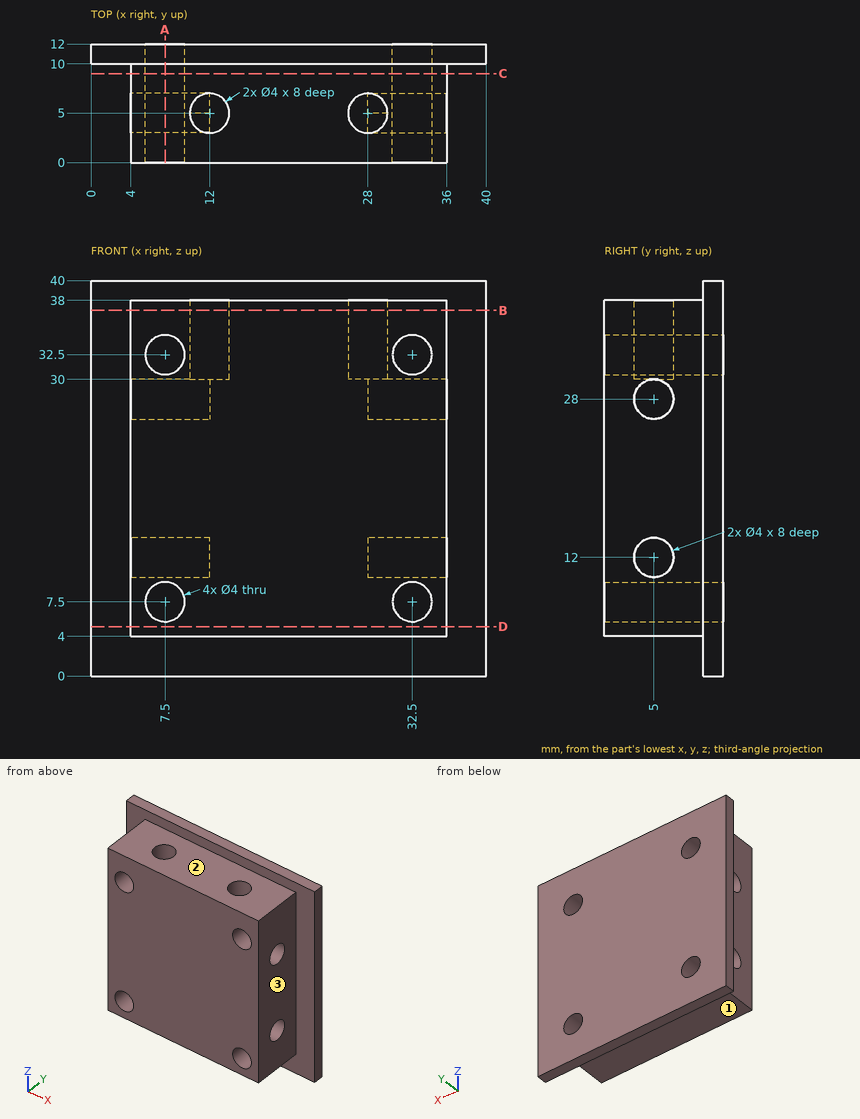
Design review of the part shown in the three views and the two pictorial views. Dimensions are in mm from the part's minimum x, y and z. A direction names the side the tool comes from. Round coordinates to 2 decimals unless told otherwise and drop trailing zeros. Loops run counter-clockwise (first coordinate to the right, second up) from the corner with the lowest first, then second, coordinate; pieces in that order, holes last.
Q1. Insertion check: pin 1 Ø3 at (y, z) = (3.5, 29) entering from +X; pin 2 Ø6 at (x, y) = (23.5, 6) entering from -Z; pin 3 Ø3 at (x, y) = (22, 7) entering from +Z. Each pin has a flat end and moves straight along its axis. Give the tip position at first contact, or say it passes through.
Result sheet:
pin 1: stops at x = 36
pin 2: stops at z = 4
pin 3: stops at z = 38
Q2. Add section C-C on y = 9. Write out the cut boundary in (x, z), plus the area to 3 significant figures.
Result sheet:
outline: (4, 4) - (36, 4) - (36, 38) - (4, 38) - close; hole circle Ø4 at (7.5, 7.5); hole circle Ø4 at (7.5, 32.5); hole circle Ø4 at (32.5, 7.5); hole circle Ø4 at (32.5, 32.5)
area: 1,040 mm2
Q3. Add section B-B on z = 37. Write out the cut boundary in (x, y).
Result sheet:
outline: (0, 10) - (4, 10) - (4, 0) - (36, 0) - (36, 10) - (40, 10) - (40, 12) - (0, 12) - close; hole circle Ø4 at (12, 5); hole circle Ø4 at (28, 5)
Q4. Add section D-D on z = 5. Write out the cut boundary in (x, y), plus the area to 3 significant figures.
Result sheet:
outline: (0, 10) - (4, 10) - (4, 0) - (36, 0) - (36, 10) - (40, 10) - (40, 12) - (0, 12) - close
area: 400 mm2
Q5. Machinability: for the marked faces 1, 2 and 3, which of the approach directions +Z, -Z, +X, -X, +Y, -Y give a long, thin tool a straight path to every point of the face, cutting with its end or side? Answer none if there is none.
Result sheet:
face 1: -Z, +X, -X, -Y
face 2: +Z, +X, -X, -Y
face 3: +Z, -Z, +X, -Y
Q6. Add section A-A on x = 7.5. Write out the cut boundary in (y, z), plus the area to 3 significant figures.
Result sheet:
outline: (0, 4) - (10, 4) - (10, 0) - (12, 0) - (12, 5.5) - (0, 5.5) - close; (0, 9.5) - (12, 9.5) - (12, 30.5) - (0, 30.5) - close; (0, 34.5) - (12, 34.5) - (12, 40) - (10, 40) - (10, 38) - (0, 38) - close; hole circle Ø4 at (5, 12); hole circle Ø4 at (5, 28)
area: 299 mm2
Q7. To check wall thickness, follow line 1 along X through (y, z) = (5, 36.25); line 2 along Z through (x, y) = (7.5, 2.75); line 3 along Y through (x, z) = (6.25, 12). State the ranges of each line that lie inside material, in increasing order.
Result sheet:
line 1: x = 4 to 10, 14 to 26, 30 to 36
line 2: z = 4 to 5.5, 9.5 to 30.5, 34.5 to 38
line 3: y = 0 to 3, 7 to 12
